Input: dimensioned drawing with shaded views. Units: mm. Origin: part minimum x, y, z. Round coordinates to 2 decimals unless told otherwise and drop trailing zeros. Order: outer loops, then holes, each group sorted by start corner. A loop starts at its lowest first (then second) coordinate and runs counter-clockwise, first axis right, second up. Notation, with made-up numbers: (-32, -36.75) - (-20, -36.75) arc R32 cw to (-20, -7.75) - close; hole circle Ø3 at (-21.75, 9). An arc over 180 degrees is marked (long way). One line per item, written item: value. Start each with the question number.
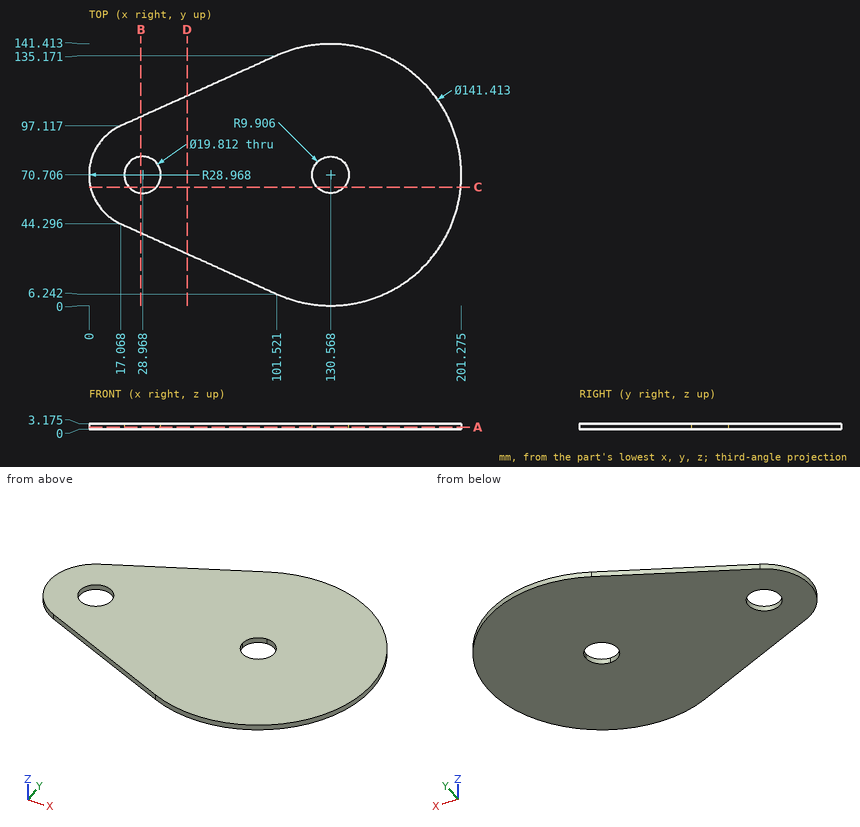
1. Line query: line 1 (X direction, y = 67, z = 2) (1 decimal); line 2 (Y direction, x = 154.5, z = 0.75); line 3 (Y direction, x = 165, z = 2). Output: solid intervals per line, ascending. Write a range as from..to.
2. Section C-C (y = 64). Return the cut outline in (x, z) (1 decimal).
3. Section D-D (x = 53). Return the cut outline in (y, z) (1 decimal).
4. Section A-A (z = 1.3). Return the cut outline in (x, y) (1 decimal).
5. Section B-B (x = 28). Return the cut outline in (y, z) (1 decimal).
6. Pin query (flat end, axial travel): pin 1 (1.5 mm diameter, centred on x = 176.5, z = 0.5, fed in from -Y); pin 2 (1 mm diameter, centred on y = 54, z = 2, fed in from -X). Return the tip coordinate at first contact, or that it passes through.
Solved:
1. line 1: x = 0.2..19.8, 38.2..121.4, 139.8..201.2
1. line 2: y = 4.17..137.24
1. line 3: y = 8.95..132.46
2. outline: (0.8, 0) - (21.7, 0) - (21.7, 3.2) - (0.8, 3.2) - close; (36.3, 0) - (123.3, 0) - (123.3, 3.2) - (36.3, 3.2) - close; (137.9, 0) - (201, 0) - (201, 3.2) - (137.9, 3.2) - close
3. outline: (28.1, 0) - (113.3, 0) - (113.3, 3.2) - (28.1, 3.2) - close
4. outline: (17.1, 44.3) - (101.5, 6.2) arc R70.7 ccw (long way) to (101.5, 135.2) - (17.1, 97.1) arc R29 ccw to start; hole circle Ø19.8 at (29, 70.7); hole circle Ø19.8 at (130.6, 70.7)
5. outline: (39.4, 0) - (60.8, 0) - (60.8, 3.2) - (39.4, 3.2) - close; (80.6, 0) - (102, 0) - (102, 3.2) - (80.6, 3.2) - close
6. pin 1: stops at y = 16.32
6. pin 2: stops at x = 4.96
